```python
from build123d import *

# Parameters (mm, degrees)
SKETCH1_W                 = 85.999999704
SKETCH1_H                 = 94.234
BOSS_EXTRUDE1_DEPTH       = 4.999999906
SKETCH2_W                 = 7.62
SKETCH2_H                 = 7.62
BOSS_EXTRUDE2_DEPTH       = 6.35
F_4_40_TAPPED_HOLE1_D     = 2.2606
F_4_40_TAPPED_HOLE1_DEPTH = 4.7498
F_4_40_TAPPED_HOLE1_TIP   = 0.679152758
F_4_CLEARANCE_HOLE1_D     = 3.2639


with BuildPart() as part:
    # Sketch1 → Boss-Extrude1 (new body)
    with BuildSketch(Plane.XY):
        Rectangle(SKETCH1_W, SKETCH1_H)
    extrude(amount=BOSS_EXTRUDE1_DEPTH)

    # Sketch2 → Boss-Extrude2 (add)
    with BuildSketch(Plane.XY.offset(4.999999906)):
        with Locations((-7.466000054, 30.607)):
            Rectangle(SKETCH2_W, SKETCH2_H)
        with Locations((34.189999946, 30.607)):
            Rectangle(SKETCH2_W, SKETCH2_H)
        with Locations((-7.466000054, -17.907)):
            Rectangle(SKETCH2_W, SKETCH2_H)
        with Locations((34.189999946, -17.907)):
            Rectangle(SKETCH2_W, SKETCH2_H)
    extrude(amount=BOSS_EXTRUDE2_DEPTH)

    # #4-40 Tapped Hole1
    with Locations(Plane.XY.offset(11.349999906)):
        with Locations((-7.466000054, 30.607), (34.189999946, 30.607), (-7.466000054, -17.907), (34.189999946, -17.907)):
            Hole(F_4_40_TAPPED_HOLE1_D / 2, depth=F_4_40_TAPPED_HOLE1_DEPTH)
            with Locations((0, 0, -(F_4_40_TAPPED_HOLE1_DEPTH + F_4_40_TAPPED_HOLE1_TIP / 2))):  # 118° drill point
                Cone(0, F_4_40_TAPPED_HOLE1_D / 2, F_4_40_TAPPED_HOLE1_TIP, mode=Mode.SUBTRACT)

    # #4 Clearance Hole1 (through all)
    with Locations(Plane.XY.offset(4.999999906)):
        with Locations((-36.649999852, 40.767), (36.649999852, 40.767), (-36.649999852, -40.767), (36.649999852, -40.767)):
            Hole(F_4_CLEARANCE_HOLE1_D / 2)


solid = part.part
```
CAD build for the part. Positions are in the model's coordinates, mm. A direction names the side the tool comes from. Give positions to 0.01 mm unless a question says otherwise; leave off trailing zeros. Order: outer loops, then holes, each group sorted by start corner. A loop starts at its lowest first (then second) coordinate and runs counter-clockwise, first axis right, second up. Notation, with made-up numbers: M 39,-36.75 L 70,-36.75 A18 ccw 70,-21.75 Z; hole C 31.5,5 d8. An arc over 180 degrees is marked long. Put each result on its own line as item: value. Start each with the question number.
(1) Drill centre lines: line 1 along Y through (x, z) = (-36.65, 3.45); line 2 along Y through (x, z) = (34.19, 9.55); line 3 along X through (y, z) = (-40, 3.25). Where is each one in solid material? Low to high.
(2) Saw through at C-C, the plane y = 13.5. Write the cut outline in (x, z).
(3) Saw through at B-B, the plane x = -36.65. Write the cut outline in (y, z).
(4) Saw through at D-D, the plane x = -24. Write the cut outline in (y, z), then the cut area to 3 significant figures.
(5) Which spindle directions (+Z, -Z, +X, -X, +Y, -Y) get a long thin tool onto all of the face, cutting with end or side? Do faces 4 (the flat face through (-8, 26.797, 8)), 5 (the flat face through (38, 31, 8)), 6 (the flat face through (-3.656, 31, 8)). Say none if no direction does.
(6) Flat gauge pins, fed straight in: pin 1 Ø3 at (x, z) = (-6.5, 9.5) entering from -Y; pin 2 Ø5 at (y, z) = (31.5, 8) entering from -X; pin 3 Ø1.9 at (y, z) = (30.5, 7) entering from +X; pin 4 Ø2 at (x, y) = (-36.65, -40.767) entering from +Z. Where does each tip first touch, or does it go through?
(7) Mould opens along Y. For faces 1 (the flat face through (-1, 47.117, 2)), 2 (the cylindrical face through (-35.02, 40.84, 2.46)), 3 (the flat face through (30.38, -18, 8)) say: +Y half, -Y half, draft (parallel to the pull), parting line (faces both ways), or undercut.
(8) Saw through at A-A, the plane x = 36.65. Write the cut outline in (y, z), then the cut area to 3 significant figures.
Check result:
1. line 1: y = -47.12 to -42.4, -39.14 to 39.14, 42.4 to 47.12
1. line 2: y = -21.72 to -19.04, -16.78 to -14.1, 26.8 to 29.48, 31.74 to 34.42
1. line 3: x = -43 to -38.09, -35.21 to 35.21, 38.09 to 43
2. outline: M -43,0 L 43,0 L 43,5 L -43,5 Z
3. outline: M -47.12,0 L -42.4,0 L -42.4,5 L -47.12,5 Z; M -39.14,0 L 39.14,0 L 39.14,5 L -39.14,5 Z; M 42.4,0 L 47.12,0 L 47.12,5 L 42.4,5 Z
4. outline: M -47.12,0 L 47.12,0 L 47.12,5 L -47.12,5 Z
4. area: 471 mm2
5. face 4: +Z, +X, -X
5. face 5: +Z, +X, +Y, -Y
5. face 6: +Z, +Y, -Y
6. pin 1: stops at y = -21.72
6. pin 2: stops at x = -11.28
6. pin 3: stops at x = 38
6. pin 4: passes through
7. face 1: +Y half
7. face 2: undercut
7. face 3: draft
8. outline: M -47.12,0 L -42.4,0 L -42.4,5 L -47.12,5 Z; M -39.14,0 L 39.14,0 L 39.14,5 L 34.42,5 L 34.42,11.35 L 26.8,11.35 L 26.8,5 L -14.1,5 L -14.1,11.35 L -21.72,11.35 L -21.72,5 L -39.14,5 Z; M 42.4,0 L 47.12,0 L 47.12,5 L 42.4,5 Z
8. area: 535 mm2
